```python
from build123d import *

# Parameters (mm, degrees)
SKETCH_1_R               = 5
EXTRUDE_1_DEPTH          = 8
SKETCH_4_R               = 4
EXTRUDE_2_DEPTH          = 1
SKETCH_2_W               = 5.05
SKETCH_2_H               = 1.88
SKETCH_2_W_2             = 1.88
SKETCH_2_H_2             = 5.15
CUT_EXTRUDE_1_DEPTH      = 12.445523142
FILLET_1_R               = 0.6
CUT_EXTRUDE_2_DEPTH      = 0.5
CUT_EXTRUDE_2_DEPTH_BACK = 13.098786096
SKETCH_3_R               = 1.2


with BuildPart() as part:
    # ｽｹｯﾁ1 → ﾎﾞｽ - 押し出し1 (new body)
    with BuildSketch(Plane.XY):
        Circle(SKETCH_1_R)
    extrude(amount=EXTRUDE_1_DEPTH)

    # ｽｹｯﾁ4 → ﾎﾞｽ - 押し出し2 (add)
    with BuildSketch(Plane(origin=(0, 0, 0), x_dir=(-1, 0, 0), z_dir=(0, 0, -1))):
        Circle(SKETCH_4_R)
    extrude(amount=EXTRUDE_2_DEPTH)

    # ｽｹｯﾁ2 → ｶｯﾄ - 押し出し1 (cut, through all)
    with BuildSketch(Plane.XY.offset(8)):
        Rectangle(SKETCH_2_W, SKETCH_2_H)
        Rectangle(SKETCH_2_W_2, SKETCH_2_H_2)
    extrude(amount=-CUT_EXTRUDE_1_DEPTH, mode=Mode.SUBTRACT)

    # ﾌｨﾚｯﾄ1
    fillet_1_edges = [part.edges().sort_by_distance(p)[0] for p in [
        (-0.94, 0.94, 3.5),
        (0.94, -0.94, 3.5),
        (-0.94, -0.94, 3.5),
        (0.94, 0.94, 3.5),
    ]]
    fillet(fillet_1_edges, radius=FILLET_1_R)

    # ｽｹｯﾁ3 → ｶｯﾄ - 押し出し2 (cut, two sides: drawn at the far end of the back side and taken through both)
    with BuildSketch(Plane(origin=(0, -2.575, 0), x_dir=(1, 0, 0), z_dir=(0, 1, 0)).offset(-CUT_EXTRUDE_2_DEPTH_BACK)):
        with Locations(Location((0, -4, 0), (0, 0, 90))):
            Circle(SKETCH_3_R)
    extrude(amount=CUT_EXTRUDE_2_DEPTH + CUT_EXTRUDE_2_DEPTH_BACK, mode=Mode.SUBTRACT)


solid = part.part
```
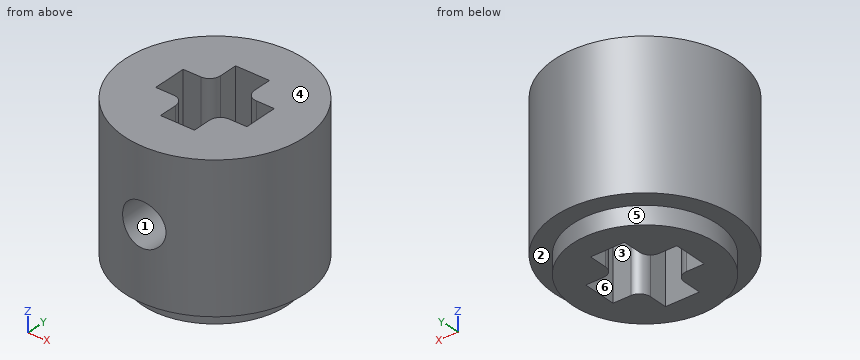
Check sheet for the modelled part. Datum: model origin and axes. Units: mm. Face numbers are marked on the shaded views. A direction names the side the tool comes from. Round coordinates to 2 decimals unless told otherwise and drop trailing zeros. Write each loop counter-clockwise with the first axis right and the second up, starting at its lowest first coordinate (ties: lowest second). Pieces come first, ordered by that corner, then holes. Notation, with made-up numbers: (81.5, 51.25) -> (105.5, 51.25) arc R12 cw to (105.5, 58.25) -> close; hole circle Ø7 at (85, -33.75). An arc over 180 degrees is marked (long way). One line per question, with ' | ' between items. Start each with the question number.
1. Set-up check for the marked faces 1, 2 and 3: record each of +Z, -Z, +X, -X, +Y, -Y from which the full face is reachable in a straight line by a thin tool's end or side.
2. Release check for a two-part mould opening along Y. For the marked faces 4, 5 and 6 record: +Y half, -Y half, draft (parallel to the pull), parting line (faces both ways), or undercut.
3. Sectioned sample at D-D, the plane x = 2.25. Record the cut outline in (y, z).
4. Scan lines: line 1 along Y through (x, z) = (0, 7.5) (3 decimals); line 2 along X through (y, z) = (-4.1, 4); line 3 along X through (y, z) = (-3, 4). Record each from-to range of solid material in increasing order. Write a range as from..to.
5. Sectioned sample at B-B, the plane z = 2. Record the cut outline in (x, y) (3 decimals).
6. Sectioned sample at C-C, the plane x = 0. Record the cut outline in (y, z) (3 decimals).
7. Depth check by flat-ended pin: pin 1 (0.6 mm diameter, centred on y = 0.5, z = 2, fed in from -X); pin 2 (0.5 mm diameter, centred on y = -2, z = 1.5, fed in from -X); pin 3 (0.6 mm diameter, centred on x = 0.5, z = 6.5, fed in from +Y). Enter the tip coordinate at first touch or a pass-through.
8. Sectioned sample at A-A, the plane y = 0. Record the cut outline in (x, z) (3 decimals), then the cut area to 4 significant figures.
Taken from the geometry:
1) face 1: -Y | face 2: -Z | face 3: +Z, -Z
2) face 4: draft | face 5: parting line | face 6: undercut
3) outline: (-4.47, 0) -> (-3.31, 0) -> (-3.31, -1) -> (-0.94, -1) -> (-0.94, 8) -> (-4.47, 8) -> close; (0.94, -1) -> (3.31, -1) -> (3.31, 0) -> (4.47, 0) -> (4.47, 8) -> (0.94, 8) -> close
4) line 1: y = -5..-2.575, 2.575..5 | line 2: x = -2.86..-1.2, 1.2..2.86 | line 3: x = -4..-1.2, 1.2..4
5) outline: circle Ø10 at (0, 0); hole (-2.525, -0.94) -> (-1.54, -0.94) arc R0.6 cw to (-0.94, -1.54) -> (-0.94, -2.575) -> (0.94, -2.575) -> (0.94, -1.54) arc R0.6 cw to (1.54, -0.94) -> (2.525, -0.94) -> (2.525, 0.94) -> (1.54, 0.94) arc R0.6 cw to (0.94, 1.54) -> (0.94, 2.575) -> (-0.94, 2.575) -> (-0.94, 1.54) arc R0.6 cw to (-1.54, 0.94) -> (-2.525, 0.94) -> close
6) outline: (-5, 0) -> (-4, 0) -> (-4, -1) -> (-2.575, -1) -> (-2.575, 2.8) -> (-5, 2.8) -> close; (-5, 5.2) -> (-2.575, 5.2) -> (-2.575, 8) -> (-5, 8) -> close; (2.575, -1) -> (4, -1) -> (4, 0) -> (5, 0) -> (5, 8) -> (2.575, 8) -> close
7) pin 1: stops at x = -5 | pin 2: stops at x = -4.68 | pin 3: stops at y = 5
8) outline: (-5, 0) -> (-4, 0) -> (-4, -1) -> (-2.525, -1) -> (-2.525, 8) -> (-5, 8) -> close; (2.525, -1) -> (4, -1) -> (4, 0) -> (5, 0) -> (5, 8) -> (2.525, 8) -> close | area: 42.55 mm^2
